Part model, mm, in its own coordinate system. A direction names the side the tool comes from. Give positions to 0.01 mm unless a question says otherwise; leave off trailing zeros. Write each loop counter-clockwise with the first axis right and the second up, starting at its lowest first coordinate (ties: lowest second). Pieces come first, ordered by that corner, then holes. Notation, with made-up numbers: (82.5, 67) - (126.5, 67) arc R20 cw to (126.5, 73) - close; hole circle Ø7 at (-11.5, 60.5). An arc over 180 degrees is marked (long way). Answer in a Markdown table with one row per item. Add a question column.
1. Band-saw the part on D-D on x = -98.5. Write the cut outline in (y, z).
2. Band-saw the part on A-A on x = -40. Write the cut outline in (y, z).
3. Pull direction Z, two halves, no side cores. Call faces 1 (the flat face through (-57, 0, -60)), 2 (the cylindrical face through (-12.91, 6.41, -55.03)), 3 (the flat face through (-55, 6, -85.69)): released by +Z, released by -Z, zero draft, split by the parting line, or undercut.
4. Band-saw the part on C-C on z = -52. Write the cut outline in (x, y).
5. Band-saw the part on B-B on y = 7.5. Write the cut outline in (x, z).
6. Which spindle directions (+Z, -Z, +X, -X, +Y, -Y) get a long thin tool onto all of the face, cutting with end or side? Do faces 4 (the flat face through (-19.18, 6, -38)), 5 (the flat face through (-57, 13, -60)). Say none if no direction does.
7. Probe line 1 along Z through (x, y) = (-100.58, 7); line 2 along X through (y, z) = (10.5, -12.5); line 3 along X through (y, z) = (11.5, -28). List the from-to ranges inside material, lowest first.
```python
from build123d import *

# Parameters (mm, degrees)
SKETCH3_R           = 8
SKETCH3_W           = 73.4
SKETCH3_H           = 33.99
BOSS_EXTRUDE1_DEPTH = 13


with BuildPart() as part:
    # Sketch3 → Boss-Extrude1 (new body)
    with BuildSketch(Plane(origin=(0, 0, 0), x_dir=(1, 0, 0), z_dir=(0, 1, 0))):
        Polygon((-121.76, 12.85), (-121.76, -10), (-108.58, -10), (-11.18, -10), (-3.18, -10), (10, -10), (10, 62.84), (10, 85.69), (-3.18, 85.69), (-11.18, 85.69), (-108.58, 85.69), (-121.76, 85.69), (-121.76, 62.84), align=None)
        with Locations((-100.58, 12.85)):
            Circle(SKETCH3_R, mode=Mode.SUBTRACT)
        with BuildLine():
            Line((-19.18, 12.85), (-19.18, 20.85))
            Line((-19.18, 20.85), (-11.18, 20.85))
            ThreePointArc((-11.18, 20.85), (-5.523145751, 18.506854249), (-3.18, 12.85))
            ThreePointArc((-3.18, 12.85), (-11.18, 4.85), (-19.18, 12.85))
        make_face(mode=Mode.SUBTRACT)
        with BuildLine():
            Line((-92.58, 54.84), (-100.58, 54.84))
            ThreePointArc((-100.58, 54.84), (-106.236854249, 68.496854249), (-92.58, 62.84))
            Line((-92.58, 62.84), (-92.58, 54.84))
        make_face(mode=Mode.SUBTRACT)
        with Locations((-55.88, 37.845)):
            Rectangle(SKETCH3_W, SKETCH3_H, mode=Mode.SUBTRACT)
        with Locations((-11.18, 62.84)):
            Circle(SKETCH3_R, mode=Mode.SUBTRACT)
        with BuildLine():
            ThreePointArc((-92.58, 62.84), (-94.923145751, 57.183145751), (-100.58, 54.84))
            Line((-100.58, 54.84), (-92.58, 54.84))
            Line((-92.58, 54.84), (-92.58, 62.84))
        make_face()
        with BuildLine():
            Line((-11.18, 20.85), (-19.18, 20.85))
            Line((-19.18, 20.85), (-19.18, 12.85))
            ThreePointArc((-19.18, 12.85), (-16.836854249, 18.506854249), (-11.18, 20.85))
        make_face()
    extrude(amount=BOSS_EXTRUDE1_DEPTH)


solid = part.part
```
Values:
| question | item | result |
|---|---|---|
| 1 | outline | (0, -85.69) - (13, -85.69) - (13, -70.56) - (0, -70.56) - close; (0, -55.12) - (13, -55.12) - (13, -20.57) - (0, -20.57) - close; (0, -5.13) - (13, -5.13) - (13, 10) - (0, 10) - close |
| 2 | outline | (0, -85.69) - (13, -85.69) - (13, -54.84) - (0, -54.84) - close; (0, -20.85) - (13, -20.85) - (13, 10) - (0, 10) - close |
| 3 | face 1 | zero draft |
| 3 | face 2 | undercut |
| 3 | face 3 | released by -Z |
| 4 | outline | (-121.76, 0) - (-92.58, 0) - (-92.58, 13) - (-121.76, 13) - close; (-19.18, 0) - (10, 0) - (10, 13) - (-19.18, 13) - close |
| 5 | outline | (-121.76, -85.69) - (10, -85.69) - (10, 10) - (-121.76, 10) - close; hole circle Ø16 at (-100.58, -62.84); hole circle Ø16 at (-100.58, -12.85); hole (-92.58, -54.84) - (-19.18, -54.84) - (-19.18, -20.85) - (-92.58, -20.85) - close; hole circle Ø16 at (-11.18, -62.84); hole circle Ø16 at (-11.18, -12.85) |
| 6 | face 4 | +Y, -Y |
| 6 | face 5 | +Z, -Z, +X, -X, +Y |
| 7 | line 1 | z = -85.69 to -70.84, -54.84 to -20.85, -4.85 to 10 |
| 7 | line 2 | x = -121.76 to -108.57, -92.59 to -19.17, -3.19 to 10 |
| 7 | line 3 | x = -121.76 to -92.58, -19.18 to 10 |
